Model file for the job. Use its own axes, mm. A direction names the side the tool comes from. Round coordinates to 2 decimals unless told otherwise and drop trailing zeros. Order: outer loops, then holes, each group sorted by start corner. A loop starts at its lowest first (then second) coordinate and runs counter-clockwise, first axis right, second up. Notation, with made-up numbers: (-35.5, -35.5) - (20.5, -35.5) arc R32 cw to (20.5, -9.5) - close; hole circle Ø11 at (71.5, 17). An arc over 180 degrees is marked (long way). Put each result on its own line as item: value. Start each with the question number.
Item 1: Pin check, flat tips, straight feed: pin 1 Ø2 at (x, z) = (2.5, 3.5) entering from -Y; pin 2 Ø4 at (y, z) = (-1.5, -0.5) entering from -X; pin 3 Ø2 at (x, z) = (-25, 2.5) entering from +Y; pin 4 Ø3 at (x, y) = (-28.5, 1.5) entering from -Z. Stop position of each tip, or through.
Item 2: Mould opens along Z. For faces 4 (the face through (-13.709, 4.247, 0.943)), 5 (the face through (6.75, 4, 3)), 6 (the face through (6.24, 6.2, 1.38)) say: pulls with the +Z half, pulls with the -Z half, needs draft (parallel to the pull), parting line crosses it, or undercut.
Item 3: Saw through at A-A on z = 0. List the corners of the cut face in (x, y).
Item 4: Which spindle directions (+Z, -Z, +X, -X, +Y, -Y) get a long thin tool onto all of the face, cutting with end or side? Do faces 1 (the face through (-35.5, -3, 0)), 2 (the face through (5.75, 5, 1)), 3 (the face through (-35, -1, 3)). Say none if no direction does.
Item 5: Saw through at C-C on x = -15.5. List the corners of the cut face in (y, z), plus the area to 3 significant figures.
Item 6: Probe probe 1 along Y at (x, z) = (-19.5, 0); probe 2 along Y at (x, z) = (-35.25, 0). List the from-to ranges inside material, lowest first.
Item 7: Saw through at D-D on z = 5.25. List the corners of the cut face in (x, y), plus the area to 3 significant figures.
```python
from build123d import *

# Parameters (mm, degrees)
SKETCH2_R           = 4.85
SKETCH2_R_2         = 2.75
BOSS_EXTRUDE1_DEPTH = 0.5
FILLET1_R           = 0.25


with BuildPart() as part:
    # Sketch1 → Revolve1 (revolve)
    with BuildSketch(Plane(origin=(0, 0, 0), x_dir=(1, 0, 0), z_dir=(0, 1, 0))):
        Polygon((-35, 4.35), (6.75, 4.35), (6.75, 6.35), (5.75, 6.35), (5.75, 4.85), (-35, 4.85), align=None)
    revolve(axis=Axis((0, 0, 0), (-1, 0, 0)))

    # Sketch2 → Boss-Extrude1 (add)
    with BuildSketch(Plane.ZY.offset(35)):
        Circle(SKETCH2_R)
        Circle(SKETCH2_R_2, mode=Mode.SUBTRACT)
    extrude(amount=BOSS_EXTRUDE1_DEPTH)

    # Fillet1
    fillet1_edges = [part.edges().sort_by_distance(p)[0] for p in [
        (-35.5, 0, -4.85),
        (-35, 0, 4.35),
    ]]
    fillet(fillet1_edges, radius=FILLET1_R)


solid = part.part
```
Results found:
1. pin 1: stops at y = -4.16
1. pin 2: stops at x = -35.5
1. pin 3: stops at y = 4.61
1. pin 4: stops at z = -4.85
2. face 4: undercut
2. face 5: needs draft
2. face 6: parting line crosses it
3. outline: (-35.5, -4.6) arc R0.25 ccw to (-35.25, -4.85) - (5.75, -4.85) - (5.75, -6.35) - (6.75, -6.35) - (6.75, -4.35) - (-34.75, -4.35) arc R0.25 cw to (-35, -4.1) - (-35, -2.75) - (-35.5, -2.75) - close; (-35.5, 2.75) - (-35, 2.75) - (-35, 4.1) arc R0.25 cw to (-34.75, 4.35) - (6.75, 4.35) - (6.75, 6.35) - (5.75, 6.35) - (5.75, 4.85) - (-35.25, 4.85) arc R0.25 ccw to (-35.5, 4.6) - close
4. face 1: +Z, -Z, -X, +Y, -Y
4. face 2: -X
4. face 3: +X
5. outline: circle Ø9.7 at (0, 0); hole circle Ø8.7 at (0, 0)
5. area: 14.5 mm²
6. probe 1: y = -4.85 to -4.35, 4.35 to 4.85
6. probe 2: y = -4.85 to -2.75, 2.75 to 4.85
7. outline: (5.75, -3.57) - (6.75, -3.57) - (6.75, 3.57) - (5.75, 3.57) - close
7. area: 7.14 mm²
